Autodesk Inventor part; units mm, degrees
ref_plane "YZ Plane" through (0, 0, 0) normal (1, 0, 0) x (0, 1, 0)
ref_plane "XZ Plane" through (0, 0, 0) normal (0, 1, 0) x (-1, 0, 0)
ref_plane "XY Plane" through (0, 0, 0) normal (0, 0, 1) x (1, 0, 0)
sketch "Sketch1" plane through (0, 0, 0) normal (0, 0, 1) x (1, 0, 0)
  line L0 (0, 83.82) -> (0, -13.97)
  line L1 (-5.4356, 0) -> (32.6136, 0)
  line L2 (0, 0) -> (27.178, 0)
  line L3 (27.178, 0) -> (27.178, 69.85)
  line L4 (27.178, 69.85) -> (0, 69.85)
  line L5 (0, 69.85) -> (0, 0)
  line L6 (0, 34.925) -> (27.178, 34.925) construction
  point P0 (5.5372, 20.6502)
  point P1 (21.59, 57.15)
  point P2 (21.59, 12.7)
  dimension "d0" = 27.178
  dimension "d1" = 69.85
  dimension "d9" = 5.588
  dimension "d10" = 22.225
  dimension "d11" = 22.225
  dimension "d29" = 21.6408
  dimension "d30" = 20.6502
extrude "Extrusion1" add sketch "Sketch1" along normal blind 5.842
hole "Hole1" at (21.59, 57.15, 0) at (21.59, 12.7, 0) direction (0, 0, 1) diameter 3.81 end through all
hole "Hole2" at (5.5372, 20.6502, 0) direction (0, 0, 1) diameter 5.3594 end through all
fillet "Fillet1" radius 6.35 2 edges at (0, 69.85, 2.921) (0, 0, 2.921)
Geometry check sheet. Reference: the model listing, model coordinates, mm. Round coordinates to 2 decimals unless told otherwise and drop trailing zeros. Order: outer loops, then holes, each group sorted by start corner. A loop starts at its lowest first (then second) coordinate and runs counter-clockwise, first axis right, second up. Notation, with made-up numbers: M 14.5,80.25 L 61.5,80.25 A31 ccw 61.5,111.25 Z; hole C 77,-2.75 d10. An arc over 180 degrees is marked long. Write item = value, one per line.
Q1. Section check D-D (y = 12.7). Enter the section's corners in (x, z) (3 decimals), plus the area to 3 significant figures.
Answer block:
outline = M 0,0 L 19.685,0 L 19.685,5.842 L 0,5.842 Z; M 23.495,0 L 27.178,0 L 27.178,5.842 L 23.495,5.842 Z
area = 137 mm^2
Q2. Depth check by flat-ended pin: pin 1 Ø4.5 at (x, y) = (5.54, 20.65) entering from -Z. Enter the tip coordinate at first touch or a pass-through.
Answer block:
pin_1 = through
Q3. Section check C-C (z = 4). Enter the section's corners in (x, y) (3 decimals).
Answer block:
outline = M 0,6.35 A6.35 ccw 6.35,0 L 27.178,0 L 27.178,69.85 L 6.35,69.85 A6.35 ccw 0,63.5 Z; hole C 5.537,20.65 d5.359; hole C 21.59,12.7 d3.81; hole C 21.59,57.15 d3.81
Q4. Section check B-B (x = 21.59). Enter the section's corners in (y, z) (3 decimals), plus the area to 3 significant figures.
Answer block:
outline = M 0,0 L 10.795,0 L 10.795,5.842 L 0,5.842 Z; M 14.605,0 L 55.245,0 L 55.245,5.842 L 14.605,5.842 Z; M 59.055,0 L 69.85,0 L 69.85,5.842 L 59.055,5.842 Z
area = 364 mm^2
Q5. Scan lines: line 1 (Y direction, x = 21.5, z = 5.1); line 2 (Y direction, x = 21, z = 4.3); line 3 (Y direction, x = 3.5, z = 1.6). Record each from-to range of solid material in increasing order.
Answer block:
line_1 = 0 to 10.8, 14.6 to 55.25, 59.05 to 69.85
line_2 = 0 to 10.89, 14.51 to 55.34, 58.96 to 69.85
line_3 = 0.68 to 18.91, 22.39 to 69.17
Q6. Section check A-A (y = 57.5). Enter the section's corners in (x, z).
Answer block:
outline = M 0,0 L 19.72,0 L 19.72,5.84 L 0,5.84 Z; M 23.46,0 L 27.18,0 L 27.18,5.84 L 23.46,5.84 Z
Q7. Release check for a two-part mould opening along X. For faces 1 (the flat face through (27.178, 34, 3)), 2 (the cylindrical face through (4.732, 23.206, 2.962)), 3 (the flat face through (13, 35, 5.842)) record: released by +X, released by -X, zero draft, split by the parting line, or undercut.
Answer block:
face_1 = released by +X
face_2 = undercut
face_3 = zero draft
